Autodesk Inventor part; units mm, degrees
ref_plane "YZ Plane" through (0, 0, 0) normal (1, 0, 0) x (0, 1, 0)
ref_plane "XZ Plane" through (0, 0, 0) normal (0, 1, 0) x (-1, 0, 0)
ref_plane "XY Plane" through (0, 0, 0) normal (0, 0, 1) x (1, 0, 0)
sketch "Sketch1" plane through (0, 0, 0) normal (0, 0, 1) x (1, 0, 0)
  line L0 (0, 0) -> (0, 4)
  line L1 (0, 4) -> (0.36, 4)
  line L2 (0.36, 4) -> (2.36, 2)
  line L3 (2.36, 2) -> (8, 2)
  line L4 (8, 2) -> (8, 0)
  line L5 (8, 0) -> (0, 0)
  dimension "d0" = 4
  dimension "d1" = 0.36
  dimension "d2" = 135
  dimension "d3" = 8
  dimension "d4" = 2
revolve "Revolution1" add sketch "Sketch1" angle 360 about axis through (8, 0, 0) along (-1, 0, 0)
chamfer "Chamfer1" distance 0.5 angle 45 1 edges at (8, -2, 0)
sketch "Sketch2" plane through (0, 0, 0) normal (-1, 0, 0) x (0, 0, 1)
  circle A0 centre (0, 0) radius 4
  line L0 (-1.4434, 0) -> (-0.7217, 1.25)
  line L1 (-0.7217, 1.25) -> (0.7217, 1.25)
  line L2 (0.7217, 1.25) -> (1.4434, 0)
  line L3 (1.4434, 0) -> (0.7217, -1.25)
  line L4 (0.7217, -1.25) -> (-0.7217, -1.25)
  line L5 (-0.7217, -1.25) -> (-1.4434, 0)
  dimension "d9" = 2.5
extrude "Extrusion1" cut sketch "Sketch2" against normal blind 1.5 contours L0 L1 L2 L3 L4 L5
thread "Thread1"
properties part number "FHS4x8" material "Steel, Alloy"
Model file for the job. Use its own axes, mm. A direction names the side the tool comes from. Coordinates: 2 decimals unless noted, no trailing zeros. Write each loop counter-clockwise with the first axis right and the second up, starting at its lowest first coordinate (ties: lowest second). Pieces come first, ordered by that corner, then holes. Notation, with made-up numbers: (31.5, 20.25) -> (81.5, 20.25) arc R28 cw to (81.5, 42.25) -> close; hole circle Ø2 at (-37.5, -28). An arc over 180 degrees is marked (long way). One line per item, written item: value. Start each with the question number.
1) Pull direction Y, two halves, no side cores. Call faces 1 (the face through (1.5, 0, 0)), 2 (the face through (0.74, 0.616, -1.088)), 3 (the face through (0.183, -0.867, -3.905)), 4 (the face through (8, 0, 0)): +Y half, -Y half, draft (parallel to the pull), parting line (faces both ways), or undercut.
2) Which spindle directions (+Z, -Z, +X, -X, +Y, -Y) get a long thin tool onto all of the face, cutting with end or side? Do faces 5 (the face through (0.74, -0.616, 1.088)), 6 (the face through (5, 0, -2)), 7 (the face through (0, 2, 0)). Say none if no direction does.
3) Slice it at A-A on z = 0. Write the cut outline in (x, y).
4) Slice it at B-B on x = 2.75. Write the cut outline in (y, z), then the cut area to 3 significant figures.
5) Flat gauge pins, fed straight in: pin 1 Ø2 at (x, y) = (1, 1) entering from -Z; pin 2 Ø1.3 at (y, z) = (0.5, 0) entering from -X; pin 3 Ø1 at (x, z) = (1.5, -1.5) entering from +Y. Where does each tip first touch, or does it go through?
6) Probe probe 1 along X at (y, z) = (3.25, -1.75); probe 2 along Y at (x, z) = (1, -1.5); probe 3 along Z at (x, y) = (6, -0.5). List the from-to ranges inside material, lowest first.
Answers follow:
1. face 1: undercut
1. face 2: undercut
1. face 3: parting line
1. face 4: draft
2. face 5: -X
2. face 6: +X
2. face 7: +Z, -Z, -X, +Y, -Y
3. outline: (0, -4) -> (0.36, -4) -> (2.36, -2) -> (7.5, -2) -> (8, -1.5) -> (8, 1.5) -> (7.5, 2) -> (2.36, 2) -> (0.36, 4) -> (0, 4) -> (0, 1.25) -> (1.5, 1.25) -> (1.5, -1.25) -> (0, -1.25) -> close
4. outline: circle Ø4 at (0, 0)
4. area: 12.6 mm2
5. pin 1: z = -3.99
5. pin 2: x = 1.5
5. pin 3: y = 3.05
6. probe 1: 0 to 0.67
6. probe 2: -3.01 to 3.01
6. probe 3: -1.94 to 1.94
